Part model, mm, in its own coordinate system. Give positions to 0.01 mm unless a question says otherwise; leave off trailing zeros. Write each loop counter-clockwise with the first axis right and the second up, starting at its lowest first coordinate (ties: lowest second). Pieces come first, ordered by that corner, then holes.
```python
from build123d import *

# Parameters (mm, degrees)
SKETCH_1_W            = 8
SKETCH_1_H            = 7.5
EXTRUDE_1_DEPTH       = 10
CHAMFER_1_SIZE        = 0.5
HOLE_WIZARD_4_0_4_1_D = 4


with BuildPart() as part:
    # 草图1 → 凸台-拉伸1 (new, symmetric)
    with BuildSketch(Plane.XY):
        Rectangle(SKETCH_1_W, SKETCH_1_H)
    extrude(amount=EXTRUDE_1_DEPTH, both=True)

    # 倒角1
    chamfer_1_edges = [part.edges().sort_by_distance(p)[0] for p in [
        (4, 0, 10),
        (-4, 0, 10),
        (4, 0, -10),
        (-4, 0, -10),
    ]]
    chamfer(chamfer_1_edges, length=CHAMFER_1_SIZE)

    # Ø4.0 (4) 直径孔1 (through all)
    with Locations(Plane(origin=(51.8, -3.75, -33), x_dir=(-1, 0, 0), z_dir=(0, -1, 0))):
        with Locations((51.965, -38), (51.965, -28)):
            Hole(HOLE_WIZARD_4_0_4_1_D / 2)


solid = part.part
```
1) Two-plate mould, pull along Z, no slides. Class faces 1 (the face through (-0.599, 0.053, 6.952)), 2 (the face through (0, 0, -10)), 3 (the face through (0, 0, 10)), 4 (the face through (0, -3.75, 0)): +Z half, -Z half, draft (parallel to the pull), parting line (faces both ways), or undercut.
Answers follow:
face 1: undercut
face 2: -Z half
face 3: +Z half
face 4: draft
2) Pin check, flat tips, straight feed: pin 1 Ø3.5 at (x, z) = (-0.165, -5) entering from +Y; pin 2 Ø4.5 at (x, z) = (-0.165, 5) entering from +Y. Stop position of each tip, or through.
Answers follow:
pin 1: passes through
pin 2: stops at y = 3.75
3) Saw through at B-B, the plane y = 1. Write the cut outline in (x, z) (3 decimals), then the cut area to 3 significant figures.
Answers follow:
outline: (-4, -9.5) - (-3.5, -10) - (3.5, -10) - (4, -9.5) - (4, 9.5) - (3.5, 10) - (-3.5, 10) - (-4, 9.5) - close; hole circle Ø4 at (-0.165, -5); hole circle Ø4 at (-0.165, 5)
area: 134 mm2
4) Wall check: L1, parallel to Z at x = 0.25, y = -2; L2, parallel to Z at x = -0.75, y = -0.5; L3, parallel to X at y = -0.75, z = 4.5. Give the ranges that are in metal, low to high.
Answers follow:
L1: z = -10 to -6.96, -3.04 to 3.04, 6.96 to 10
L2: z = -10 to -6.91, -3.09 to 3.09, 6.91 to 10
L3: x = -4 to -2.1, 1.77 to 4
5) Saw through at C-C, the plane x = -1.5. Write the cut outline in (y, z), then the cut area to 3 significant figures.
Answers follow:
outline: (-3.75, -10) - (3.75, -10) - (3.75, -6.49) - (-3.75, -6.49) - close; (-3.75, -3.51) - (3.75, -3.51) - (3.75, 3.51) - (-3.75, 3.51) - close; (-3.75, 6.49) - (3.75, 6.49) - (3.75, 10) - (-3.75, 10) - close
area: 105 mm2
6) Saw through at A-A, the plane z = 5. Write the cut outline in (x, y) (3 decimals), then the cut area to 3 significant figures.
Answers follow:
outline: (-4, -3.75) - (-2.165, -3.75) - (-2.165, 3.75) - (-4, 3.75) - close; (1.835, -3.75) - (4, -3.75) - (4, 3.75) - (1.835, 3.75) - close
area: 30.0 mm2
7) Saw through at D-D, the plane z = -6.5. Write the cut outline in (x, y), then the cut area to 3 significant figures.
Answers follow:
outline: (-4, -3.75) - (-1.49, -3.75) - (-1.49, 3.75) - (-4, 3.75) - close; (1.16, -3.75) - (4, -3.75) - (4, 3.75) - (1.16, 3.75) - close
area: 40.2 mm2
